Drawing for the job (mm, zero at the part's lowest x, y, z). A direction names the side the tool comes from. Round coordinates to 2 decimals unless told otherwise and drop trailing zeros. Loops run counter-clockwise (first coordinate to the right, second up) from the corner with the lowest first, then second, coordinate; pieces in that order, holes last. Notation, with made-up numbers: (52.25, 50.25) -> (78.25, 50.25) arc R23 cw to (78.25, 69.25) -> close; hole circle Ø5 at (39.25, 74). An arc over 180 degrees is marked (long way). Put each result on its own line as item: value. Start each with the question number.
Item 1: Cut at C-C, the plane x = 53. List the corners of the cut face in (y, z), plus the area to 3 significant figures.
Item 2: Flat gauge pins, fed straight in: pin 1 Ø6 at (y, z) = (226.5, 46) entering from -X; pin 2 Ø10 at (y, z) = (194.5, 31) entering from +X. Where does each tip first touch, or does it go through?
Item 3: Cut at B-B, the plane z = 28.5. List the corners of the cut face in (x, y).
Item 4: Cut at A-A, the plane y = 256. List the corners of the cut face in (x, z), plus the area to 3 significant figures.
Item 5: Tool access for the marked faces 1 and 2: list every direction of +Z, -Z, +X, -X, +Y, -Y with a clear straight run to the whole face (end or side of a thin tool).
Item 6: Drill centre lines: probe 1 along Z at (x, y) = (22, 208); probe 2 along X at (y, z) = (59.5, 8.5). Where is each one in solid material? Low to high. Write a range as [from, to].
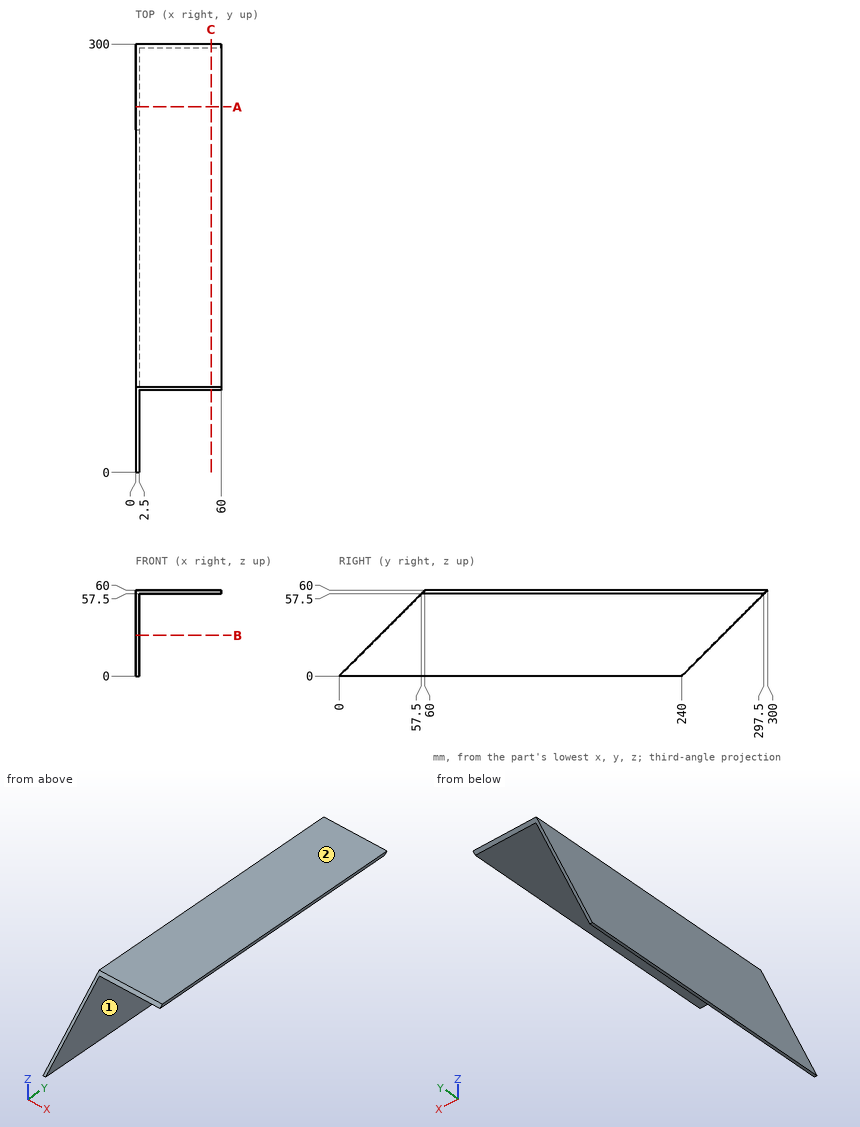
Reply:
1. outline: (57.5, 57.5) -> (297.5, 57.5) -> (300, 60) -> (60, 60) -> close
1. area: 600 mm^2
2. pin 1: stops at x = 0
2. pin 2: stops at x = 2.5
3. outline: (0, 28.5) -> (2.5, 28.5) -> (2.5, 268.5) -> (0, 268.5) -> close
4. outline: (0, 16) -> (2.5, 16) -> (2.5, 57.5) -> (60, 57.5) -> (60, 60) -> (0, 60) -> close
4. area: 254 mm^2
5. face 1: -Z, +X, +Y, -Y
5. face 2: +Z, +X, -X, +Y, -Y
6. probe 1: z = [57.5, 60]
6. probe 2: x = [0, 2.5]
